Read the model definition and answer for the solid it produces. Units are mm, in the model's axes. Face numbers are marked on the shaded views. A direction names the side the tool comes from. Coordinates: 2 decimals unless noted, no trailing zeros. Loops run counter-clockwise (first coordinate to the right, second up) from the corner with the lowest first, then second, coordinate; pieces in that order, holes last.
Q1. Section A-A (x = 5) is taken. Give the vertices of the cut face in (y, z), then the cut area to 3 significant figures.
Q2. Straight lines are drawn through the part: line 1 (Z direction, x = -29.6, y = -55); line 2 (Y direction, x = -4, z = 20); line 3 (X direction, y = -45.5, z = 17). For each, find the intervals that lie inside material, in ascending order.
Q3. Section B-B (y = -15) is taken. Give the vertices of the cut face in (x, z).
Q4. Flat-ended cylindrical pins translate along their axes: P1, Ø2, axis at x = -21.5, z = 4, coming from the -Y side; P2, Ø4, axis at y = -0.5, z = 15.5, coming from the +X side; P3, Ø1.5, axis at x = -6.5, z = 6, coming from the -Y side. Find the tip coordinate at first contact, or state that the pin passes through.
Q5. Section D-D (z = 19.75) is taken. Give the vertices of the cut face in (x, y), then the cut area to 3 significant figures.
Q6. Which of the six approach directions +Z, -Z, +X, -X, +Y, -Y give full straight-line access (tool end or side, diameter ignored) to the marked faces 1 and 2?
Q7. Section C-C (z = 12.5) is taken. Give the vertices of the cut face in (x, y).
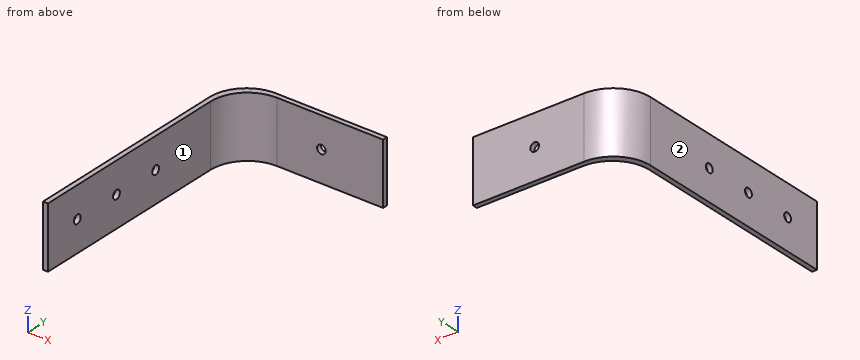
from build123d import *

# Parameters (mm, degrees)
BOSS_EXTRUDE1_DEPTH = 25
SKETCH2_R           = 1.75
CUT_EXTRUDE1_DEPTH  = 2
SKETCH3_R           = 1.75
CUT_EXTRUDE2_DEPTH  = 2


with BuildPart() as part:
    # Sketch1 → Boss-Extrude1 (new body)
    with BuildSketch(Plane.XY):
        with BuildLine():
            Line((-15, 30), (30, 30))
            Line((30, 30), (30, 28))
            Line((30, 28), (-13, 28))
            ThreePointArc((-13, 28), (-23.606601718, 23.606601718), (-28, 13))
            Line((-28, 13), (-28, -70))
            Line((-28, -70), (-30, -70))
            Line((-30, -70), (-30, 15))
            ThreePointArc((-30, 15), (-25.606601718, 25.606601718), (-15, 30))
        make_face()
    extrude(amount=BOSS_EXTRUDE1_DEPTH)

    # Sketch2 → Cut-Extrude1 (cut)
    with BuildSketch(Plane.ZY.offset(30)):
        with Locations(Location((12.5, -15, 0), (0, 0, 270))):
            Circle(SKETCH2_R)
        with Locations(Location((12.5, -35, 0), (0, 0, 270))):
            Circle(SKETCH2_R)
        with Locations(Location((12.5, -55, 0), (0, 0, 270))):
            Circle(SKETCH2_R)
    extrude(amount=-CUT_EXTRUDE1_DEPTH, mode=Mode.SUBTRACT)

    # Sketch3 → Cut-Extrude2 (cut)
    with BuildSketch(Plane(origin=(0, 30, 0), x_dir=(1, 0, 0), z_dir=(0, 1, 0))):
        with Locations(Location((5, -12.5, 0), (0, 0, 270))):
            Circle(SKETCH3_R)
    extrude(amount=-CUT_EXTRUDE2_DEPTH, mode=Mode.SUBTRACT)


solid = part.part
Numbers:
1. outline: (28, 0) - (30, 0) - (30, 10.75) - (28, 10.75) - close; (28, 14.25) - (30, 14.25) - (30, 25) - (28, 25) - close
1. area: 43.0 mm2
2. line 1: z = 0 to 10.75, 14.25 to 25
2. line 2: y = 28 to 30
2. line 3: x = -30 to -28
3. outline: (-30, 0) - (-28, 0) - (-28, 10.75) - (-30, 10.75) - close; (-30, 14.25) - (-28, 14.25) - (-28, 25) - (-30, 25) - close
4. P1: stops at y = 24.61
4. P2: stops at x = -28
4. P3: stops at y = 28
5. outline: (-30, -70) - (-28, -70) - (-28, 13) arc R15 cw to (-13, 28) - (30, 28) - (30, 30) - (-15, 30) arc R15 ccw to (-30, 15) - close
5. area: 316 mm2
6. face 1: +Z, -Z, +X, -Y
6. face 2: +Z, -Z, -X, +Y, -Y
7. outline: (-30, -70) - (-28, -70) - (-28, -56.75) - (-30, -56.75) - close; (-30, -53.25) - (-28, -53.25) - (-28, -36.75) - (-30, -36.75) - close; (-30, -33.25) - (-28, -33.25) - (-28, -16.75) - (-30, -16.75) - close; (-30, -13.25) - (-28, -13.25) - (-28, 13) arc R15 cw to (-13, 28) - (3.25, 28) - (3.25, 30) - (-15, 30) arc R15 ccw to (-30, 15) - close; (6.75, 28) - (30, 28) - (30, 30) - (6.75, 30) - close
